Geometry check sheet. Reference: the model listing, model coordinates, mm. Round coordinates to 2 decimals unless told otherwise and drop trailing zeros. Use one line per item in the form item = value. Start each with the question number.
1. Go/stop test with flat-tipped pins: pin 1 (12 mm diameter, centred on x = 326, y = -304.5, fed in from -Z); pin 2 (10 mm diameter, centred on x = 358, z = 1470.5, fed in from -Y). Record where each tip stops, or that it passes through.
2. Material ranges on line 1 (Y direction, x = 432.5, z = 1013.5); line 2 (Z direction, x = 193.5, y = -288); line 3 (X direction, y = -398.5, z = 852.5), recorded low to high.
3. Draft check along X on faces 1 (the flat face through (404, 0, 923)), 2 (the flat face through (0, -281, 897)), 3 (the flat face through (397, -170, 993)), 4 (the flat face through (820, -281, 897)). Enter one of: pulls with the +X half, pulls with the -X half, needs draft (parallel to the pull), parting line crosses it, or undercut.
```python
from build123d import *

# Parameters (mm, degrees)
F0_W     = 820
F0_H     = 1820
F1_DEPTH = 570
F2_W     = 680
F2_H     = 1500
F3_DEPTH = 400
F3_TAPER = -3


with BuildPart() as f1:
    # F0 (on Front) → F1 (new body)
    with BuildSketch(Plane.XZ):
        with Locations((410, 910)):
            Rectangle(F0_W, F0_H)
    extrude(amount=F1_DEPTH)

    # F2 (on face) → F3 (cut)
    with BuildSketch(Plane.XZ.offset(570)):
        with Locations((410, 1000)):
            Rectangle(F2_W, F2_H)
    extrude(amount=-F3_DEPTH, taper=F3_TAPER, mode=Mode.SUBTRACT)


solid = f1.part
```
Reported:
q1.pin_1 = 0
q1.pin_2 = -170
q2.line_1 = -170 to 0
q2.line_2 = 0 to 235.22, 1764.78 to 1820
q2.line_3 = 0 to 61.01, 758.99 to 820
q3.face_1 = needs draft
q3.face_2 = pulls with the -X half
q3.face_3 = undercut
q3.face_4 = pulls with the +X half
